Check sheet for the modelled part. Datum: model origin and axes. Units: mm. Face numbers are marked on the shaded views. A direction names the side the tool comes from. Round coordinates to 2 decimals unless told otherwise and drop trailing zeros. Order: outer loops, then holes, each group sorted by start corner. A loop starts at its lowest first (then second) coordinate and runs counter-clockwise, first axis right, second up. Notation, with made-up numbers: (3, -39) -> (7, -39) arc R13 ccw to (7, -33) -> close; hole circle Ø7 at (-6.5, -36). An arc over 180 degrees is marked (long way). Answer in a Markdown table with one row per item. Add a question column.
1. Sectioned sample at C-C, the plane y = 67. Record the boundary of the cut face in (x, z) (3 decimals), then the cut area to 3 significant figures.
2. Material ranges on L1, parallel to Y at x = 11, z = 1; L2, parallel to Y at x = 11.35, z = 0.5; L3, parallel to Z at x = 5, y = 72, recorded low to high. Write a range as from..to.
3. Sectioned sample at A-A, the plane y = 54.5. Record the boundary of the cut face in (x, z) (3 decimals), then the cut area to 3 significant figures.
4. Sectioned sample at B-B, the plane x = -6. Record the boundary of the cut face in (y, z) (1 decimal).
5. Access from +Z, -Z, +X, -X, +Y, -Y to the whole of each face (thin tool, end or side, straight path). Record for the marked faces 1 and 2.
6. Depth check by flat-ended pin: P1, Ø6, axis at y = 19, z = -5, coming from the -X side; P2, Ø1.4, axis at x = 1.5, z = 1, coming from the -Y side (3 decimals); P3, Ø1.4, axis at y = 45.5, z = 1, coming from the -X side; P4, Ø5.5, axis at x = 1.35, y = 11.477, coming from the -Z side. Enter the tip coordinate at first touch or a pass-through.
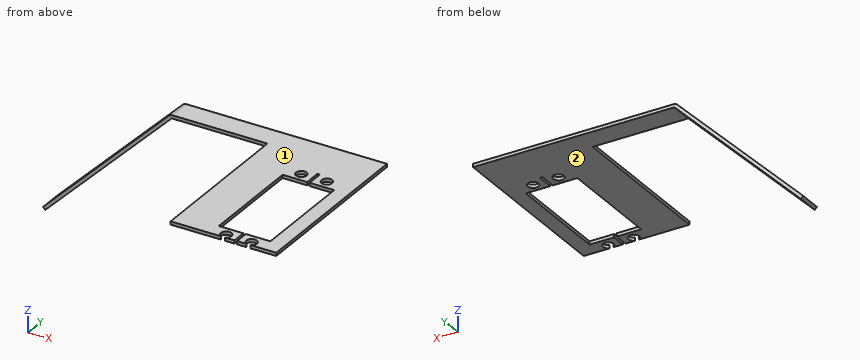
```python
from build123d import *

# Parameters (mm, degrees)
BASE_FLANGE1_DEPTH      = 9.525
BASE_FLANGE1_DEPTH_BACK = 61.9125
SKETCH9_W               = 88.097631615
SKETCH9_H               = 62.483000002
CUT_EXTRUDE1_DEPTH      = 144.762808626
SKETCH12_R              = 2.099999991
CUT_EXTRUDE2_DEPTH      = 144.762808626


# Sheet-metal steps are written as plain solids
with BuildPart() as part:
    # Sketch2 → Base-Flange1 (new, two sides: drawn at the far end of the back side and taken through both)
    with BuildSketch(Plane(origin=(0, 71.4375, 0), x_dir=(1, 0, 0), z_dir=(0, 1, 0)).offset(-BASE_FLANGE1_DEPTH_BACK)):
        with BuildLine():
            Line((-106.452002215, 49.610155888), (-57.057591472, 0.215745145))
            ThreePointArc((-57.057591472, 0.215745145), (-56.818621234, 0.056070336), (-56.536736617, 0))
            Line((-56.536736617, 0), (22.225, 0))
            Line((22.225, 0), (22.225, -1.27))
            Line((22.225, -1.27), (-56.536736617, -1.27))
            ThreePointArc((-56.536736617, -1.27), (-57.304629193, -1.11725667), (-57.955617084, -0.682280467))
            Line((-57.955617084, -0.682280467), (-107.350027828, 48.712130276))
            Line((-107.350027828, 48.712130276), (-106.452002215, 49.610155888))
        make_face()
    extrude(amount=BASE_FLANGE1_DEPTH + BASE_FLANGE1_DEPTH_BACK)

    # Sketch9 → Cut-Extrude1 (cut, through all)
    with BuildSketch(Plane.XY.offset(1.27)):
        with Locations((-63.301212021, 40.766500001)):
            Rectangle(SKETCH9_W, SKETCH9_H)
    extrude(amount=-CUT_EXTRUDE1_DEPTH, mode=Mode.SUBTRACT)

    # Sketch12 → Cut-Extrude2 (cut, through all)
    with BuildSketch(Plane.XY.offset(1.27)):
        with Locations((11.350000033, 11.477000033)):
            Circle(SKETCH12_R)
        with Locations((1.349999967, 11.477000033)):
            Circle(SKETCH12_R)
        with Locations((11.350000033, 60.077000115)):
            Circle(SKETCH12_R)
        with Locations((1.349999967, 60.077000115)):
            Circle(SKETCH12_R)
        Polygon((6.85, 8.59600008), (5.85, 8.59600008), (5.85, 15.20000008), (-3.776999939, 15.20000008), (-3.776999939, 56.354000068), (5.85, 56.354000068), (5.85, 62.958000068), (6.85, 62.958000068), (6.85, 56.354000068), (16.476999939, 56.354000068), (16.476999939, 15.20000008), (6.85, 15.20000008), align=None)
    extrude(amount=-CUT_EXTRUDE2_DEPTH, mode=Mode.SUBTRACT)


solid = part.part
```
Answer key:
| question | item | result |
|---|---|---|
| 1 | outline | (-19.252, 0) -> (22.225, 0) -> (22.225, 1.27) -> (-19.252, 1.27) -> close |
| 1 | area | 52.7 mm² |
| 2 | L1 | y = 13.55..15.2, 56.35..58.01, 62.15..80.96 |
| 2 | L2 | y = 13.58..15.2, 56.35..57.98, 62.18..80.96 |
| 2 | L3 | z = 0..1.27 |
| 3 | outline | (-19.252, 0) -> (-3.777, 0) -> (-3.777, 1.27) -> (-19.252, 1.27) -> close; (16.477, 0) -> (22.225, 0) -> (22.225, 1.27) -> (16.477, 1.27) -> close |
| 3 | area | 27.0 mm² |
| 4 | outline | (9.5, 0) -> (81, 0) -> (81, 1.3) -> (9.5, 1.3) -> close |
| 5 | face 1 | +Z, +X, -X, +Y, -Y |
| 5 | face 2 | -Z, +X, +Y, -Y |
| 6 | P1 | passes through |
| 6 | P2 | stops at y = 9.525 |
| 6 | P3 | stops at x = -19.25 |
| 6 | P4 | stops at z = 0 |
